Design review of the part built by this model. Coordinates are the model's own, in mm. Face numbers are marked on the shaded views. A direction names the side the tool comes from. Round coordinates to 2 decimals unless told otherwise and drop trailing zeros. Order: outer loops, then holes, each group sorted by start corner. A loop starts at its lowest first (then second) coordinate and runs counter-clockwise, first axis right, second up. Notation, with made-up numbers: M -18,-26.75 L -3,-26.75 A24 cw -3,-5.75 Z; hole C 55.25,43 d4. An arc over 180 degrees is marked long. Use a Markdown table: item, result. Add a question column.
(1) Take a section at D-D (z = 8). Write out the cut boundary in (x, y).
(2) To check wall thickness, follow probe 1 along Y at (x, z) = (0, 98); probe 2 along Y at (x, z) = (101.6, 36.5); probe 3 along Z at (x, y) = (-4.5, -15). State the ranges of each line that lie inside material, in increasing order. Write a range as from..to.
(3) For pin 1 (24.5 mm diameter, centred on x = 108, y = 2, fed in from +Z); pin 2 (5 mm diameter, centred on y = -6.5, z = 44.5, fed in from +X); pin 3 (5 mm diameter, centred on y = -3, z = 67, fed in from -X); pin 4 (8 mm diameter, centred on x = 87, y = -15.5, fed in from -Z), all flat-tipped, find the tip position at first contact; note any pin that passes through.
(4) Take a section at A-A (z = 75.5). Write out the cut boundary in (x, y), then the cut area to 3 significant figures.
(5) Take a section at B-B (x = 101.6). Write out the cut boundary in (y, z), then the cut area to 3 significant figures.
(6) The part is to be moulded in two halves that separate along X. For the marked faces 1, 2 and 3, say which applies: released by +X, released by -X, zero draft, split by the parting line, or undercut.
(7) Machinability: for the marked faces 4, 5 and 6, which of the approach directions +Z, -Z, +X, -X, +Y, -Y give a long, thin tool a straight path to every point of the face, cutting with its end or side? Answer none if there is none.
(8) Take a section at C-C (x = 0). Write out the cut boundary in (y, z).
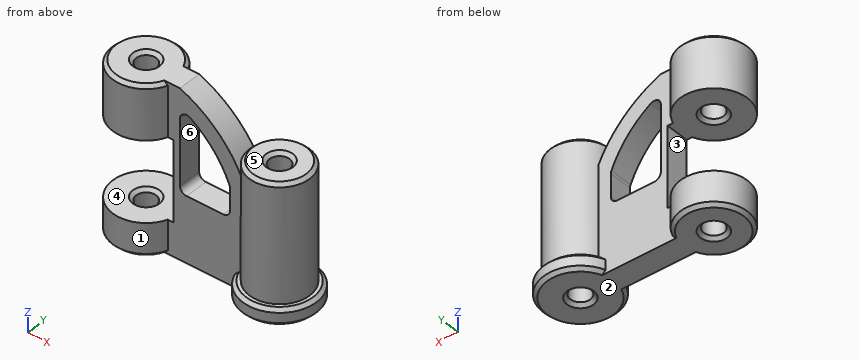
```python
from build123d import *

# Parameters (mm, degrees)
F0_R      = 25.4
F0_R_2    = 7.62
F1_DEPTH  = 127
F0_R_3    = 22.86
F2_DEPTH  = 101.6
F4_DEPTH  = 8.89
F5_W      = 60.96
F5_H      = 60.96
F6_DEPTH  = 50.8
F7_R      = 5.08
F8_SIZE   = 2.54
F9_R      = 27.94
F9_R_2    = 22.86
F10_DEPTH = 12.7
F11_SIZE  = 2.54


with BuildPart() as f1:
    # F0 (on Top) → F1 (new body)
    with BuildSketch(Plane.XY):
        Circle(F0_R)
        Circle(F0_R_2, mode=Mode.SUBTRACT)
    extrude(amount=F1_DEPTH)



with BuildPart() as f2:
    # F0 (on Top) → F2 (new body)
    with BuildSketch(Plane.XY):
        with Locations((101.6, 0)):
            Circle(F0_R_3)
        with Locations((101.6, 0)):
            Circle(F0_R_2, mode=Mode.SUBTRACT)
    extrude(amount=F2_DEPTH)


with BuildPart() as f1_1:
    add(f1.part)

    add(f2.part)  # F4 merges F2
    # F3 (on Front) → F4 (join, symmetric)
    with BuildSketch(Plane.XZ):
        with BuildLine():
            Line((20.32, 127), (20.32, 0))
            Line((20.32, 0), (81.28, 0))
            Line((81.28, 0), (81.28, 81.28))
            ThreePointArc((81.28, 81.28), (61.5844056789, 108.82076155), (33.02, 127))
            Line((33.02, 127), (20.32, 127))
        make_face()
        with BuildLine():
            ThreePointArc((33.02, 113.1692568198), (55.8815349001, 96.5627163287), (71.12, 72.7674195988))
            Line((71.12, 72.7674195988), (71.12, 49.6692568198))
            Line((71.12, 49.6692568198), (33.02, 49.6692568198))
            Line((33.02, 49.6692568198), (33.02, 113.1692568198))
        make_face(mode=Mode.SUBTRACT)
    extrude(amount=F4_DEPTH, both=True)

    # F5 (on Front) → F6 (cut, symmetric)
    with BuildSketch(Plane.XZ):
        with Locations((-2.54, 55.88)):
            Rectangle(F5_W, F5_H)
    extrude(amount=F6_DEPTH, both=True, mode=Mode.SUBTRACT)

    # F7
    f7_edges = [f1_1.edges().sort_by_distance(p)[0] for p in [
        (33.02, 0, 113.169257),
        (33.02, 0, 49.669257),
        (71.12, 0, 49.669257),
        (71.12, 0, 72.76742),
    ]]
    fillet(f7_edges, radius=F7_R)

    # F8
    f8_edges = [f1_1.edges().sort_by_distance(p)[0] for p in [
        (-25.4, 0, 127),
        (-7.62, 0, 127),
        (-7.62, 0, 25.4),
        (-25.4, 0, 0),
        (-7.62, 0, 86.36),
        (-7.62, 0, 0),
    ]]
    chamfer(f8_edges, length=F8_SIZE)

    # F9 (on Top) → F10 (join)
    with BuildSketch(Plane.XY):
        with Locations((101.6, 0)):
            Circle(F9_R)
        with Locations((101.6, 0)):
            Circle(F9_R_2, mode=Mode.SUBTRACT)
    extrude(amount=F10_DEPTH)

    # F11
    f11_edges = [f1_1.edges().sort_by_distance(p)[0] for p in [
        (93.98, 0, 0),
        (129.54, 0, 0),
        (93.98, 0, 101.6),
        (129.54, 0, 12.7),
        (78.74, 0, 101.6),
    ]]
    chamfer(f11_edges, length=F11_SIZE)


solid = f1_1.part
```
Verdict:
| question | item | result |
|---|---|---|
| 1 | outline | M 23.79,-8.89 L 75.11,-8.89 A27.94 ccw long 75.11,8.89 L 23.79,8.89 A25.4 ccw long Z; hole C 0,0 d15.24; hole C 101.6,0 d15.24 |
| 2 | probe 1 | y = -25.4..-7.62, 7.62..25.4 |
| 2 | probe 2 | y = -22.86..-7.62, 7.62..22.86 |
| 2 | probe 3 | z = 0..25.4, 86.36..127 |
| 3 | pin 1 | stops at z = 101.6 |
| 3 | pin 2 | stops at x = 124.11 |
| 3 | pin 3 | stops at x = 27.94 |
| 3 | pin 4 | stops at z = 0 |
| 4 | outline | M 27.94,-8.89 L 33.02,-8.89 L 33.02,8.89 L 27.94,8.89 Z; M 69.96,-8.89 L 80.54,-8.89 A22.86 ccw long 80.54,8.89 L 69.96,8.89 Z; hole C 101.6,0 d15.24 |
| 4 | area | 1,720 mm^2 |
| 5 | outline | M -27.94,2.54 L -25.4,0 L -10.16,0 L -7.62,2.54 L -7.62,99.06 L -10.16,101.6 L -20.32,101.6 L -22.86,99.06 L -22.86,12.7 L -25.4,12.7 L -27.94,10.16 Z; M 7.62,2.54 L 10.16,0 L 25.4,0 L 27.94,2.54 L 27.94,10.16 L 25.4,12.7 L 22.86,12.7 L 22.86,99.06 L 20.32,101.6 L 10.16,101.6 L 7.62,99.06 Z |
| 5 | area | 3,190 mm^2 |
| 6 | face 1 | undercut |
| 6 | face 2 | zero draft |
| 6 | face 3 | released by -X |
| 7 | face 4 | -X, +Y, -Y |
| 7 | face 5 | +Z, +X, +Y, -Y |
| 7 | face 6 | +Y, -Y |
| 8 | outline | M -25.4,2.54 L -22.86,0 L -10.16,0 L -7.62,2.54 L -7.62,22.86 L -10.16,25.4 L -25.4,25.4 Z; M -25.4,86.36 L -10.16,86.36 L -7.62,88.9 L -7.62,124.46 L -10.16,127 L -22.86,127 L -25.4,124.46 Z; M 7.62,2.54 L 10.16,0 L 22.86,0 L 25.4,2.54 L 25.4,25.4 L 10.16,25.4 L 7.62,22.86 Z; M 7.62,88.9 L 10.16,86.36 L 25.4,86.36 L 25.4,124.46 L 22.86,127 L 10.16,127 L 7.62,124.46 Z |
